Could you check a few things on this drawing? It's one solid part, dimensions in mm from its lowest x, y, z. Coordinates: 2 decimals unless noted, no trailing zeros. Write each loop counter-clockwise with the first axis right and the second up, starting at its lowest first coordinate (ties: lowest second). Pieces come first, ordered by that corner, then holes. Notation, with made-up numbers: M 44.5,31.5 L 101.5,31.5 A25 cw 101.5,58.5 Z; hole C 49.5,-24 d9. An arc over 180 degrees is marked long. Use a Markdown table: item, result.
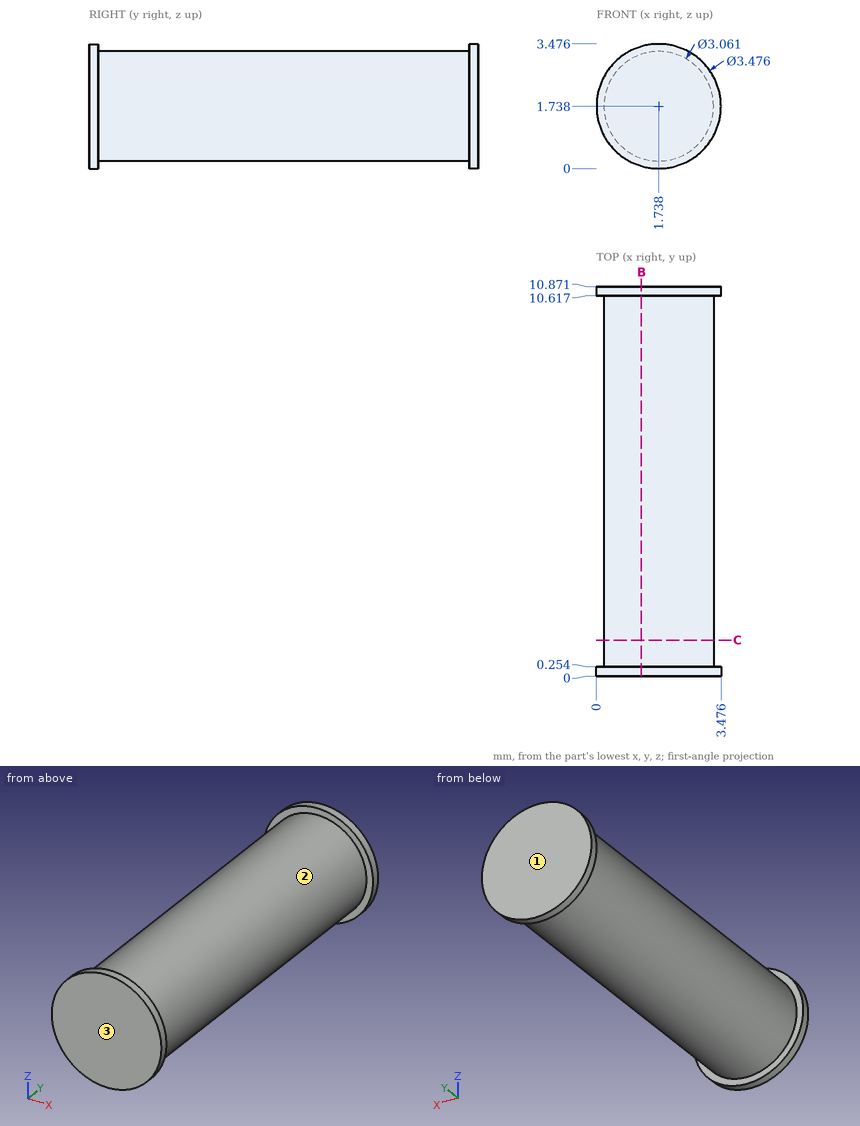
1. Suppose I cut it at C-C on y = 1. Write out the boundary of the cut face in (x, z).
Answers follow:
| item | result |
|---|---|
| outline | C 1.74,1.74 d3.06 |
2. Will these pins go through, and if not, where does the flat tip stop? pin 1 Ø1.7 at (x, z) = (2.5, 1.5) entering from -Y; pin 2 Ø2 at (y, z) = (6, 2) entering from +X.
Answers follow:
| item | result |
|---|---|
| pin 1 | stops at y = 0 |
| pin 2 | stops at x = 3.27 |
3. Suppose I cut it at B-B on x = 1.25. Write out the boundary of the cut face in (y, z).
Answers follow:
| item | result |
|---|---|
| outline | M 0,0.07 L 0.25,0.07 L 0.25,0.29 L 10.62,0.29 L 10.62,0.07 L 10.87,0.07 L 10.87,3.41 L 10.62,3.41 L 10.62,3.19 L 0.25,3.19 L 0.25,3.41 L 0,3.41 Z |
4. I need wall thicknesses on probe 1 along Y at (x, z) = (3.3, 1.75); probe 2 along X at (y, z) = (9.5, 1.8); probe 3 along Z at (x, y) = (0.9, 8). Which ranges of each line are inside material? Lowest first, please.
Answers follow:
| item | result |
|---|---|
| probe 1 | y = 0 to 0.25, 10.62 to 10.87 |
| probe 2 | x = 0.21 to 3.27 |
| probe 3 | z = 0.46 to 3.02 |
5. We'd pull the mould along Y, two halves only. Please class the marked faces 1, 2 and 3: +Y half, -Y half, draft (parallel to the pull), parting line (faces both ways), or undercut.
Answers follow:
| item | result |
|---|---|
| face 1 | +Y half |
| face 2 | undercut |
| face 3 | -Y half |
